from build123d import *

# Parameters (mm, degrees)
SKETCH_1_R          = 1.75
EXTRUDE_1_DEPTH     = 5
CUT_EXTRUDE_1_REACH = 7
SKETCH_2_W          = 35
SKETCH_2_H          = 3


with BuildPart() as part:
    # 草圖1 → 填料-伸長1 (new body)
    with BuildSketch(Plane.XY):
        Polygon((-30, 17.5), (-30, 9.5), (-22, 9.5), (-22, -9.5), (-30, -9.5), (-30, -17.5), (30, -17.5), (30, -9.5), (22, -9.5), (22, 9.5), (30, 9.5), (30, 17.5), align=None)
        with Locations((-26, 13.5)):
            Circle(SKETCH_1_R, mode=Mode.SUBTRACT)
        with Locations((26, 13.5)):
            Circle(SKETCH_1_R, mode=Mode.SUBTRACT)
        with Locations((-26, -13.5)):
            Circle(SKETCH_1_R, mode=Mode.SUBTRACT)
        with Locations((26, -13.5)):
            Circle(SKETCH_1_R, mode=Mode.SUBTRACT)
    extrude(amount=EXTRUDE_1_DEPTH)

    # 草圖2 → 除料-伸長1 (cut, up to next)
    with BuildSketch(Plane.XY.offset(5), mode=Mode.PRIVATE) as cut_extrude_1_sk1:
        with Locations((0, -8)):
            Rectangle(SKETCH_2_W, SKETCH_2_H)
    cut_extrude_1_tool1 = extrude(cut_extrude_1_sk1.sketch, amount=-CUT_EXTRUDE_1_REACH, mode=Mode.PRIVATE) & part.part
    add(cut_extrude_1_tool1.solids().sort_by_distance((0, -8, 5))[0], mode=Mode.SUBTRACT)


solid = part.part
Build history of the part. All positions in model axes, mm. A direction names the side the tool comes from. Round coordinates to 2 decimals unless told otherwise and drop trailing zeros. Loops run counter-clockwise (first coordinate to the right, second up) from the corner with the lowest first, then second, coordinate; pieces in that order, holes last. Notation, with made-up numbers: (82.25, -37) -> (119.25, -37) arc R14 cw to (119.25, -29) -> close; hole circle Ø8 at (-33, 37). An arc over 180 degrees is marked (long way). Answer in a Markdown table with one row per item.
Item 1: Saw through at D-D (x = -26). Write the cut outline in (y, z).
Answers below:
| item | result |
|---|---|
| outline | (-17.5, 0) -> (-15.25, 0) -> (-15.25, 5) -> (-17.5, 5) -> close; (-11.75, 0) -> (-9.5, 0) -> (-9.5, 5) -> (-11.75, 5) -> close; (9.5, 0) -> (11.75, 0) -> (11.75, 5) -> (9.5, 5) -> close; (15.25, 0) -> (17.5, 0) -> (17.5, 5) -> (15.25, 5) -> close |
Item 2: Saw through at B-B (x = -11.5). Write the cut outline in (y, z).
Answers below:
| item | result |
|---|---|
| outline | (-17.5, 0) -> (-9.5, 0) -> (-9.5, 5) -> (-17.5, 5) -> close; (-6.5, 0) -> (17.5, 0) -> (17.5, 5) -> (-6.5, 5) -> close |
Item 3: Saw through at A-A (z = 4.3). Write the cut outline in (x, y), and give its area (3 significant figures).
Answers below:
| item | result |
|---|---|
| outline | (-30, -17.5) -> (30, -17.5) -> (30, -9.5) -> (22, -9.5) -> (22, 9.5) -> (30, 9.5) -> (30, 17.5) -> (-30, 17.5) -> (-30, 9.5) -> (-22, 9.5) -> (-22, -9.5) -> (-30, -9.5) -> close; hole circle Ø3.5 at (-26, -13.5); hole circle Ø3.5 at (-26, 13.5); hole (-17.5, -9.5) -> (17.5, -9.5) -> (17.5, -6.5) -> (-17.5, -6.5) -> close; hole circle Ø3.5 at (26, -13.5); hole circle Ø3.5 at (26, 13.5) |
| area | 1,650 mm² |
Item 4: Mould opens along X. For faces 1 (the flat face through (17.5, -8, 3)), 2 (the flat face through (30, 13, 2)), 3 (the flat face through (0, 0, 5)) say: +X half, -X half, draft (parallel to the pull), parting line (faces both ways), or undercut.
Answers below:
| item | result |
|---|---|
| face 1 | undercut |
| face 2 | +X half |
| face 3 | draft |
Item 5: Which spindle directions (+Z, -Z, +X, -X, +Y, -Y) get a long thin tool onto all of the face, cutting with end or side? Do faces 4 (the flat face through (0, -17.5, 2)), 5 (the flat face through (-17.5, -8, 3)), 6 (the flat face through (26, -9.5, 2)), 7 (the flat face through (-26, 9.5, 2)). Say none if no direction does.
Answers below:
| item | result |
|---|---|
| face 4 | +Z, -Z, +X, -X, -Y |
| face 5 | +Z, -Z |
| face 6 | +Z, -Z, +X |
| face 7 | +Z, -Z, -X |
Item 6: Drill centre lines: L1, parallel to Y at x = -26, z = 3.55; L2, parallel to Y at x = 22.5, z = 0.45; L3, parallel to X at y = -7.5, z = 2.35. Where is each one in solid material? Low to high. Write a range as [from, to].
Answers below:
| item | result |
|---|---|
| L1 | y = [-17.5, -15.25], [-11.75, -9.5], [9.5, 11.75], [15.25, 17.5] |
| L2 | y = [-17.5, -9.5], [9.5, 17.5] |
| L3 | x = [-22, -17.5], [17.5, 22] |
Item 7: Saw through at C-C (y = -13.5). Write the cut outline in (x, z).
Answers below:
| item | result |
|---|---|
| outline | (-30, 0) -> (-27.75, 0) -> (-27.75, 5) -> (-30, 5) -> close; (-24.25, 0) -> (24.25, 0) -> (24.25, 5) -> (-24.25, 5) -> close; (27.75, 0) -> (30, 0) -> (30, 5) -> (27.75, 5) -> close |
Item 8: Pin check, flat tip, straight feed: pin 1 (0.9 mm diameter, centred on y = -8.5, z = 2.5, fed in from +X). Stop position of the tip, or through.
Answers below:
| item | result |
|---|---|
| pin 1 | stops at x = 22 |
